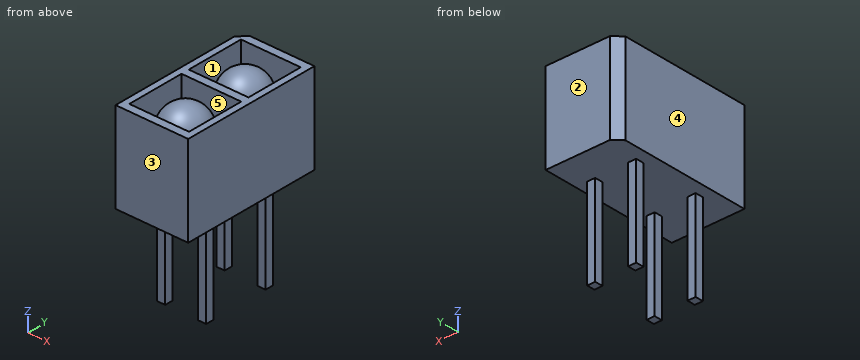
Autodesk Inventor part; units mm, degrees
ref_plane "YZ Plane" through (0, 0, 0) normal (1, 0, 0) x (0, 1, 0)
ref_plane "XZ Plane" through (0, 0, 0) normal (0, 1, 0) x (-1, 0, 0)
ref_plane "XY Plane" through (0, 0, 0) normal (0, 0, 1) x (1, 0, 0)
sketch "スケッチ1" plane through (0, 0, 0) normal (0, 0, 1) x (1, 0, 0)
  line L0 (-2.25, 4.35) -> (2.25, 4.35)
  line L1 (2.25, 4.35) -> (2.25, -4.35)
  line L2 (2.25, -4.35) -> (-2.25, -4.35)
  line L3 (-2.25, -4.35) -> (-2.25, 4.35)
  line L4 (-3.4568, 2.05) -> (3.4568, 2.05) construction
  line L5 (3.4568, -2.05) -> (-3.4568, -2.05) construction
  line L6 (-4.4106, 0) -> (4.4106, 0) construction
  line L7 (-1.85, 3.85) -> (1.85, 3.85)
  line L8 (1.85, 3.85) -> (1.85, 0.25)
  line L9 (1.85, 0.25) -> (-1.85, 0.25)
  line L10 (-1.85, 0.25) -> (-1.85, 3.85)
  line L11 (-1.85, -0.25) -> (1.85, -0.25)
  line L12 (1.85, -0.25) -> (1.85, -3.85)
  line L13 (1.85, -3.85) -> (-1.85, -3.85)
  line L14 (-1.85, -3.85) -> (-1.85, -0.25)
  line L15 (-1.75, 4.35) -> (-2.25, 3.85)
  circle A0 centre (0, 2.05) radius 1.45
  circle A1 centre (0, -2.05) radius 1.45
  line L16 (1.27, 5.4107) -> (1.27, -6.214) construction
  line L17 (-1.27, -6.214) -> (-1.27, 5.4107) construction
  line L18 (0, 6.0924) -> (0, -6.0924) construction
  line L19 (1.52, 2.3) -> (1.02, 2.3)
  line L20 (1.02, 2.3) -> (1.02, 1.8)
  line L21 (1.02, 1.8) -> (1.52, 1.8)
  line L22 (1.52, 1.8) -> (1.52, 2.3)
  line L23 (-1.02, 2.3) -> (-1.52, 2.3)
  line L24 (-1.52, 2.3) -> (-1.52, 1.8)
  line L25 (-1.52, 1.8) -> (-1.02, 1.8)
  line L26 (-1.02, 1.8) -> (-1.02, 2.3)
  line L27 (1.52, -1.8) -> (1.02, -1.8)
  line L28 (1.02, -1.8) -> (1.02, -2.3)
  line L29 (1.02, -2.3) -> (1.52, -2.3)
  line L30 (1.52, -2.3) -> (1.52, -1.8)
  line L31 (-1.02, -1.8) -> (-1.52, -1.8)
  line L32 (-1.52, -1.8) -> (-1.52, -2.3)
  line L33 (-1.52, -2.3) -> (-1.02, -2.3)
  line L34 (-1.02, -2.3) -> (-1.02, -1.8)
  point P0 (0, 0)
  point P1 (0, 4.35)
  point P2 (-2.25, 0)
  point P3 (0, 0)
  point P4 (-1.85, 2.05)
  point P5 (0, 3.85)
  point P6 (1.85, -2.05)
  point P7 (0, -3.85)
  point P8 (1.27, 2.3)
  point P9 (1.52, 2.05)
  point P10 (-1.27, 2.3)
  point P11 (-1.52, 2.05)
  point P12 (1.27, -1.8)
  point P13 (1.52, -2.05)
  point P14 (-1.27, -1.8)
  dimension "d0" = 4.5
  dimension "d1" = 8.7
  dimension "d2" = 4.1
  dimension "d3" = 3.7
  dimension "d4" = 3.6
  dimension "d5" = 0.5
  dimension "d6" = 0.5
  dimension "d9" = 2.9
  dimension "d13" = 2.54
  dimension "d14" = 0.5
extrude "押し出し1" add sketch "スケッチ1" along normal blind 5.6 contours L0 L1 L2 L3 L15
extrude "押し出し2" add sketch "スケッチ1" along normal blind 5.6 contours A0 L21 L20 L19 | L19 L20 L21 A0 L25 L26 L23 | L23 L26 L25 A0 | A1 L29 L28 L27 | L27 L28 L29 A1 L33 L34 L31 | L31 L34 L33 A1
fillet "フィレット1" radius 1.45 2 edges at (-1.45, 2.05, 5.6) (-1.45, -2.05, 5.6)
extrude "押し出し3" add sketch "スケッチ1" against normal blind 5.6 contours A0 L21 L20 L19 | A0 L19 L22 L21 | L23 L26 L25 A0 | A0 L25 L24 L23 | A1 L29 L28 L27 | A1 L27 L30 L29 | L31 L34 L33 A1 | A1 L33 L32 L31
extrude "押し出し4" add sketch "スケッチ1" along normal blind 0.5 contours L7 L8 L9 L10 | L11 L12 L13 L14 | A0 L21 L20 L19 | A0 L19 L22 L21 | L19 L20 L21 A0 L25 L26 L23 | L23 L26 L25 A0 | A0 L25 L24 L23 | A1 L29 L28 L27 | A1 L27 L30 L29 | L27 L28 L29 A1 L33 L34 L31 | L31 L34 L33 A1 | A1 L33 L32 L31
equation "\"d6\" = d5"
properties part number "LBR-127"
Model file for the job. Use its own axes, mm. Face numbers are marked on the shaded views. A direction names the side the tool comes from. Coordinates: 2 decimals unless noted, no trailing zeros. Write each loop counter-clockwise with the first axis right and the second up, starting at its lowest first coordinate (ties: lowest second). Pieces come first, ordered by that corner, then holes. Notation, with made-up numbers: (5, -11.5) - (19, -11.5) arc R14 cw to (19, -4.5) - close; hole circle Ø1 at (23, 43). An arc over 180 degrees is marked (long way). Use a Markdown table: item, result. Add a question column.
Item 1: Band-saw the part on A-A, the plane z = 4. Write the cut outline in (x, y).
Item 2: Band-saw the part on D-D, the plane x = -0.35. Write the cut outline in (y, z).
Item 3: Band-saw the part on B-B, the plane z = -2.5. Write the cut outline in (x, y).
Item 4: Two-plate mould, pull along Y, no slides. Class the marked faces 3, 4 and 5: pulls with the +Y half, pulls with the -Y half, needs draft (parallel to the pull), parting line crosses it, or undercut.
Item 5: Drop flat-ended pins along their axis: pin 1 (1 mm diameter, centred on y = -1.5, z = -1.5, fed in from -X); pin 2 (1.1 mm diameter, centred on x = -1, y = 2.5, fed in from +Z); pin 3 (0.6 mm diameter, centred on x = 1.5, z = -2, fed in from +Y). Give the stop position or say it passes through.
Item 6: Drill centre lines: line 1 along X through (y, z) = (-3, 1.5); line 2 along X through (y, z) = (-0.5, 4); line 3 along Y through (x, z) = (-0.75, 4.25). Where is each one in solid material? Low to high.
Item 7: Band-saw the part on C-C, the plane y = 2.05. Write the cut outline in (x, z).
Item 8: 3-axis set-ups, long thin cutter, end or side, ignore diameter. For the marked faces 1 and 2: which of +Z, -Z, +X, -X, +Y, -Y reach the whole face in a straight line?
A:
| question | item | result |
|---|---|---|
| 1 | outline | (-2.25, -4.35) - (2.25, -4.35) - (2.25, 4.35) - (-1.75, 4.35) - (-2.25, 3.85) - close; circle Ø2.9 at (0, -2.05); circle Ø2.9 at (0, 2.05); hole (-1.85, -3.85) - (1.85, -3.85) - (1.85, -0.25) - (-1.85, -0.25) - close; hole (-1.85, 0.25) - (1.85, 0.25) - (1.85, 3.85) - (-1.85, 3.85) - close |
| 2 | outline | (-4.35, 0) - (4.35, 0) - (4.35, 5.6) - (3.85, 5.6) - (3.85, 0.5) - (3.46, 0.5) - (3.46, 4.15) arc R1.41 ccw to (0.64, 4.15) - (0.64, 0.5) - (0.25, 0.5) - (0.25, 5.6) - (-0.25, 5.6) - (-0.25, 0.5) - (-0.64, 0.5) - (-0.64, 4.15) arc R1.41 ccw to (-3.46, 4.15) - (-3.46, 0.5) - (-3.85, 0.5) - (-3.85, 5.6) - (-4.35, 5.6) - close |
| 3 | outline | (-1.52, -2.3) - (-1.02, -2.3) - (-1.02, -1.8) - (-1.52, -1.8) - close; (-1.52, 1.8) - (-1.02, 1.8) - (-1.02, 2.3) - (-1.52, 2.3) - close; (1.02, -2.3) - (1.52, -2.3) - (1.52, -1.8) - (1.02, -1.8) - close; (1.02, 1.8) - (1.52, 1.8) - (1.52, 2.3) - (1.02, 2.3) - close |
| 4 | face 3 | pulls with the -Y half |
| 4 | face 4 | needs draft |
| 4 | face 5 | undercut |
| 5 | pin 1 | stops at x = -1.52 |
| 5 | pin 2 | stops at z = 5.49 |
| 5 | pin 3 | stops at y = 2.3 |
| 6 | line 1 | x = -2.25 to -1.85, -1.1 to 1.1, 1.85 to 2.25 |
| 6 | line 2 | x = -2.25 to -1.85, 1.85 to 2.25 |
| 6 | line 3 | y = -4.35 to -3.85, -3.29 to -0.81, -0.25 to 0.25, 0.81 to 3.29, 3.85 to 4.35 |
| 7 | outline | (-2.25, 0) - (-1.52, 0) - (-1.52, -5.6) - (-1.02, -5.6) - (-1.02, 0) - (1.02, 0) - (1.02, -5.6) - (1.52, -5.6) - (1.52, 0) - (2.25, 0) - (2.25, 5.6) - (1.85, 5.6) - (1.85, 0.5) - (1.45, 0.5) - (1.45, 4.15) arc R1.45 ccw to (-1.45, 4.15) - (-1.45, 0.5) - (-1.85, 0.5) - (-1.85, 5.6) - (-2.25, 5.6) - close |
| 8 | face 1 | +Z |
| 8 | face 2 | +Z, -Z, +X, -X, +Y |
